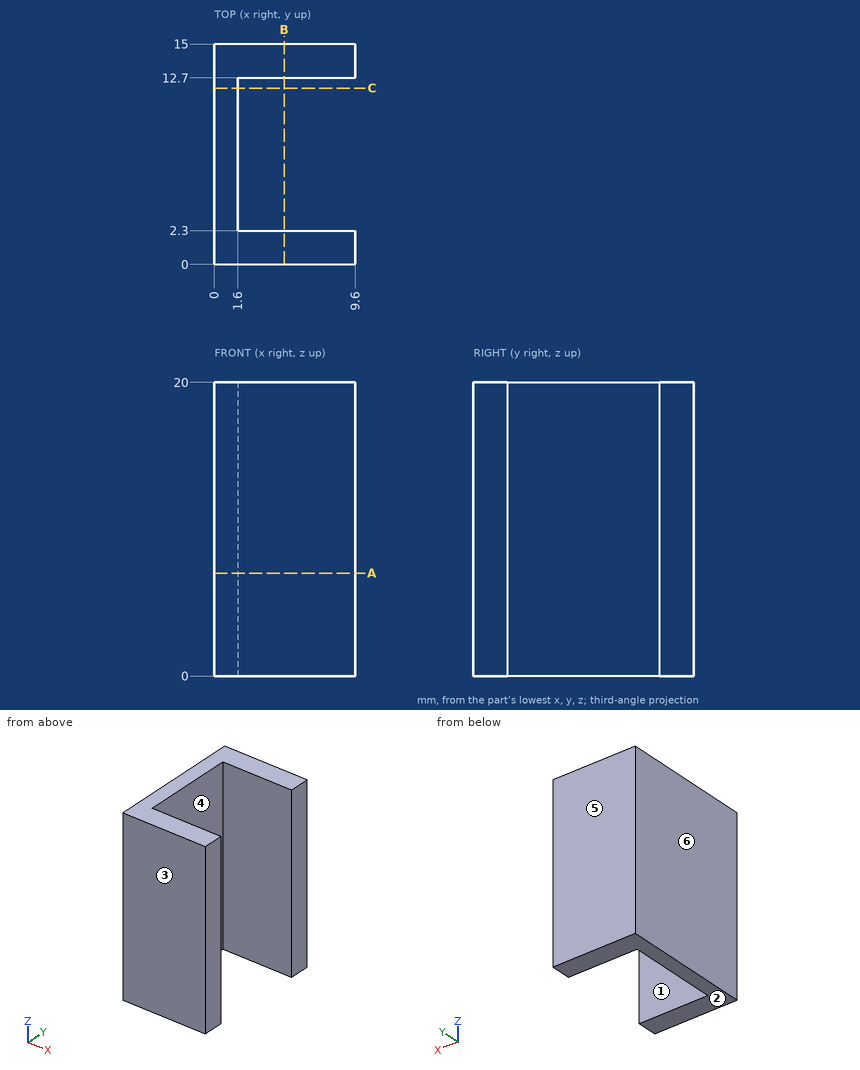
Job drawing, mm, ordinate dimensions from the low corner. One solid piece. A direction names the side the tool comes from. Coordinates: 2 decimals unless noted, no trailing zeros. Order: outer loops, then holes, each group sorted by start corner. A loop starts at its lowest first (then second) coordinate and runs counter-clockwise, first axis right, second up. Notation, with made-up numbers: M -27,65 L 31,65 A13 ccw 31,75 Z; hole C -31.5,-5.75 d5. An arc over 180 degrees is marked long. Answer as CSV lines item,"result".
(1) Band-saw the part on C-C, the plane y = 12. List the corners of the cut face in (x, z), then the cut area to 3 significant figures.
Geometry says:
outline,"M 0,0 L 1.6,0 L 1.6,20 L 0,20 Z"
area,"32.0 mm2"
(2) Band-saw the part on B-B, the plane x = 4.75. List the corners of the cut face in (y, z), then the cut area to 3 significant figures.
Geometry says:
outline,"M 0,0 L 2.3,0 L 2.3,20 L 0,20 Z; M 12.7,0 L 15,0 L 15,20 L 12.7,20 Z"
area,"92.0 mm2"
(3) Band-saw the part on A-A, the plane z = 7. List the corners of the cut face in (x, y), then the cut area to 3 significant figures.
Geometry says:
outline,"M 0,0 L 9.6,0 L 9.6,2.3 L 1.6,2.3 L 1.6,12.7 L 9.6,12.7 L 9.6,15 L 0,15 Z"
area,"60.8 mm2"
(4) Wall check: line 1 along Y through (x, z) = (6.75, 13.5); line 2 along X through (y, z) = (5, 3.5). Give the ranges that are in metal, low to high.
Geometry says:
line 1,"y = 0 to 2.3, 12.7 to 15"
line 2,"x = 0 to 1.6"
(5) Pull direction Y, two halves, no side cores. Call the marked faces 3, 4, 5 and 6: +Y half, -Y half, draft (parallel to the pull), parting line (faces both ways), or undercut.
Geometry says:
face 3,"-Y half"
face 4,"undercut"
face 5,"+Y half"
face 6,"draft"
(6) 3-axis set-ups, long thin cutter, end or side, ignore diameter. For the marked faces 1 and 2: which of +Z, -Z, +X, -X, +Y, -Y reach the whole face in a straight line?
Geometry says:
face 1,"+Z, -Z, +X"
face 2,"-Z, +X, -X, +Y, -Y"
